```python
from build123d import *

# Parameters (mm, degrees)
CROQUIS1_R              = 8.5
SALIENTE_EXTRUIR1_DEPTH = 4.6
CROQUIS6_R              = 6.35
CORTAR_EXTRUIR1_DEPTH   = 13.870897405
CROQUIS13_R             = 2.775
CORTAR_EXTRUIR7_DEPTH   = 10
SALIENTE_EXTRUIR4_DEPTH = 4.6
SALIENTE_EXTRUIR6_DEPTH = 10
CHAFL_N1_SIZE           = 3
REDONDEO1_R             = 1
CROQUIS16_R             = 1
CORTAR_EXTRUIR8_DEPTH   = 5
CHAFL_N3_SIZE           = 3
REDONDEO3_R             = 1
CROQUIS19_R             = 1
CORTAR_EXTRUIR10_DEPTH  = 5
CROQUIS20_R             = 1
CORTAR_EXTRUIR11_DEPTH  = 5


with BuildPart() as part:
    # Croquis1 → Saliente-Extruir1 (new body)
    with BuildSketch(Plane.XY):
        Circle(CROQUIS1_R)
    extrude(amount=SALIENTE_EXTRUIR1_DEPTH)

    # Croquis6 → Cortar-Extruir1 (cut, through all)
    with BuildSketch(Plane.XY.offset(4.6)):
        Circle(CROQUIS6_R)
    extrude(amount=-CORTAR_EXTRUIR1_DEPTH, mode=Mode.SUBTRACT)

    # Croquis13 → Cortar-Extruir7 (cut)
    with BuildSketch(Plane(origin=(0, 0, 0), x_dir=(-1, 0, 0), z_dir=(0, 0, -1))):
        with Locations((4.716932975, -4.100371118)):
            Circle(CROQUIS13_R)
    extrude(amount=-CORTAR_EXTRUIR7_DEPTH, mode=Mode.SUBTRACT)

    # Croquis14 → Saliente-Extruir4 (add)
    with BuildSketch(Plane(origin=(0, 0, 0), x_dir=(-1, 0, 0), z_dir=(0, 0, -1))):
        with BuildLine():
            ThreePointArc((1.551676597, -6.157499471), (7.565960492, -6.576995274), (6.313526123, -0.679623346))
            ThreePointArc((6.313526123, -0.679623346), (6.23633763, -1.196073977), (6.11697615, -1.704436205))
            ThreePointArc((6.11697615, -1.704436205), (7.102852286, -2.683326996), (7.490692392, -4.017403077))
            ThreePointArc((7.490692392, -4.017403077), (6.844195938, -5.949574331), (5.020802515, -6.858683701))
            ThreePointArc((5.020802515, -6.858683701), (3.645732845, -6.660284257), (2.539161891, -5.820236841))
            ThreePointArc((2.539161891, -5.820236841), (2.052358742, -6.0091866), (1.551676597, -6.157499471))
        make_face()
    extrude(amount=-SALIENTE_EXTRUIR4_DEPTH)

    # Croquis15 → Saliente-Extruir6 (add)
    with BuildSketch(Plane(origin=(0, 0, 0), x_dir=(-1, 0, 0), z_dir=(0, 0, -1))):
        Polygon((6.067896868, 4.315078912), (7, 2.545563795), (20.271363381, 9.536337286), (19.339260249, 11.305852404), align=None)
        Polygon((0.121525269, -22.401216868), (0.703019524, -7.412492291), (-1.295477087, -7.334959724), (-1.876971341, -22.323684301), align=None)
        Polygon((-19.460785518, 11.095364464), (-6.770916391, 3.097413379), (-5.704522913, 4.789395929), (-18.39439204, 12.787347014), align=None)
    extrude(amount=SALIENTE_EXTRUIR6_DEPTH)

    # Chaflán1
    chafl_n1_edges = [part.edges().sort_by_distance(p)[0] for p in [
        (-7.525199261, 3.952388655, 0),
    ]]
    chamfer(chafl_n1_edges, length=CHAFL_N1_SIZE)

    # Redondeo1
    redondeo1_edges = [part.edges().sort_by_distance(p)[0] for p in [
        (-19.805311815, 10.421094845, 0),
        (-6.533948434, 3.430321354, -10),
        (-19.805311815, 10.421094845, -10),
    ]]
    fillet(redondeo1_edges, radius=REDONDEO1_R)

    # Croquis16 → Cortar-Extruir8 (cut)
    with BuildSketch(Plane(origin=(-0.470783925, -0.893741523, 0), x_dir=(-0.8847575587350184, 0.46605156609676857, 0), z_dir=(-0.4660515660967685, -0.8847575587350183, 0))):
        with Locations(Location((9.379666904, 7.5, 0), (0, 0, 180))):
            Circle(CROQUIS16_R)
        with Locations(Location((19.379666904, 7.5, 0), (0, 0, 180))):
            Circle(CROQUIS16_R)
    extrude(amount=-CORTAR_EXTRUIR8_DEPTH, mode=Mode.SUBTRACT)

    # Chaflán3
    chafl_n3_edges = [part.edges().sort_by_distance(p)[0] for p in [
        (0.339730649, -8.493208056, 0),
        (7.185468612, 4.540819401, 0),
    ]]
    chamfer(chafl_n3_edges, length=CHAFL_N3_SIZE)

    # Redondeo3
    redondeo3_edges = [part.edges().sort_by_distance(p)[0] for p in [
        (0.877723036, -22.362450584, 0),
        (0.296228781, -7.373726008, -10),
        (0.877723036, -22.362450584, -10),
        (18.927588779, 11.941355739, 0),
        (6.237719652, 3.943404654, -10),
        (18.927588779, 11.941355739, -10),
    ]]
    fillet(redondeo3_edges, radius=REDONDEO3_R)

    # Croquis19 → Cortar-Extruir10 (cut)
    with BuildSketch(Plane(origin=(-0.989101784, -0.038372645, 0), x_dir=(0, 0, 1), z_dir=(-0.9992483051032128, -0.038766283654184684, 0))):
        with Locations(Location((-7.5, -9.379666904, 0), (0, 0, 270))):
            Circle(CROQUIS19_R)
        with Locations(Location((-7.5, -19.379666904, 0), (0, 0, 270))):
            Circle(CROQUIS19_R)
    extrude(amount=-CORTAR_EXTRUIR10_DEPTH, mode=Mode.SUBTRACT)

    # Croquis20 → Cortar-Extruir11 (cut)
    with BuildSketch(Plane(origin=(0.527782577, -0.83740095, 0), x_dir=(0.8459912750808336, 0.5331967390064434, 0), z_dir=(0.5331967390064434, -0.8459912750808336, 0))):
        with Locations((9.379666904, -7.5)):
            Circle(CROQUIS20_R)
        with Locations((19.379666904, -7.5)):
            Circle(CROQUIS20_R)
    extrude(amount=-CORTAR_EXTRUIR11_DEPTH, mode=Mode.SUBTRACT)


solid = part.part
```
Can you work these out from the model? Positions are in its coordinate system, mm. A direction names the side the tool comes from. Coordinates: 2 decimals unless noted, no trailing zeros. Write each loop counter-clockwise with the first axis right and the second up, starting at its lowest first coordinate (ties: lowest second). Pieces come first, ordered by that corner, then holes. Notation, with made-up numbers: M -21,69.5 L 6,69.5 A28 cw 6,99.5 Z; hole C 33,78.25 d7. An arc over 180 degrees is marked long. Write item = value, one per line. Start each with the question number.
Q1. If we section it at A-A, the plane y = 0: Write out the boundary of the cut face in (x, z).
Q2. On a 3-axis mill with a long thin cutter (end or side, diameter ignored), from which of +Z, -Z, +X, -X, +Y, -Y can I reach the whole of each face in a straight line? I mean faces 1 (the face through (-6.807, 3.558, -9.715)), 2 (the face through (7.83, 4.93, -6.51)). Say none if no direction works.
Q3. If I drill on L1, parallel to X at y = 0, z = 2.6; L2, parallel to Y at x = 1, z = 0.5; L3, parallel to X at y = 6, z = -0.25, over which ranges is the centre line in solid material (lowest first)? Write a range as [from, to].
Q4. I'm going to push flat-ended pins straight in: pin 1 (0.7 mm diameter, centred on x = 0.5, y = -18, fed in from +Z); pin 2 (4 mm diameter, centred on x = 6, z = -5, fed in from -Y); pin 3 (5 mm diameter, centred on x = -2.5, z = -0.5, fed in from +Y). Where does each tip first touch, or does it pass through?
Q5. Thinking about a two-plate mould opening in X: for faces 3 (the face through (18.681, 11.769, -0.285)), 4 (the face through (-8.83, 4.65, 1.52)), 5 (the face through (-3.628, -6.653, 2.268)), 6 (the face through (14, 9, 0)), which applies, released by +X, released by -X, zero draft, split by the parting line, or undercut?
Q6. If we section it at B-B, the plane z = -1.5: Write out the boundary of the cut face in (x, y), then the cut area to 3 significant figures.
Q7. If we section it at C-C, the plane x = 4.5: Write out the boundary of the cut face in (y, z), then the cut area to 3 significant figures.
Q8. If we section it at D-D, the plane z = 1: Write out the boundary of the cut face in (x, y) (3 decimals).
Check sheet entries:
q1.outline = M -8.5,0 L -6.35,0 L -6.35,4.6 L -8.5,4.6 Z; M 6.35,0 L 8.5,0 L 8.5,4.6 L 6.35,4.6 Z
q2.face_1 = -Z, -Y
q2.face_2 = none
q3.L1 = [-8.5, -6.35], [6.35, 8.5]
q3.L2 = [-10.95, -6.27], [6.27, 8.44]
q3.L3 = [-13.56, -9.27], [7.63, 11.38]
q4.pin_1 = 0
q4.pin_2 = 3.1
q4.pin_3 = 8.5
q5.face_3 = released by +X
q5.face_4 = released by -X
q5.face_5 = undercut
q5.face_6 = zero draft
q6.outline = M -20.27,9.54 L -7,2.55 L -6.07,4.32 L -19.34,11.31 Z; M -0.7,-7.41 L -0.12,-22.4 L 1.88,-22.32 L 1.3,-7.33 Z; M 5.7,4.79 L 6.77,3.1 L 19.46,11.1 L 18.39,12.79 Z
q6.area = 90.0 mm²
q7.outline = M -7.21,0 L -4.48,0 L -4.48,4.6 L -7.21,4.6 Z; M 4.48,0 L 7.21,0 L 7.21,4.6 L 4.48,4.6 Z
q7.area = 25.1 mm²
q8.outline = M -9.718,3.977 L -7.938,3.04 A8.5 ccw -8.129,-2.485 A3.775 ccw -3.592,-7.704 A8.5 ccw -0.662,-8.474 L -0.584,-10.484 A10.5 ccw 1.415,-10.404 L 1.337,-8.394 A8.5 ccw 7.67,3.664 L 9.371,4.736 A10.5 ccw 8.303,6.427 L 6.601,5.355 A8.5 ccw -7.008,4.81 L -8.787,5.748 A10.5 ccw Z; hole M -7.491,-4.017 A2.662 ccw -5.021,-6.859 A2.775 ccw -2.539,-5.82 A6.35 ccw long -6.117,-1.704 A2.775 ccw Z
